Answer from the drawing. Dimensions are ordinates in mm from the lowest x, y and z of the part. Give positions to 0.01 mm unless a question says otherwise; leave off trailing zeros. Write each loop counter-clockwise with the first axis right and the second up, starting at its lowest first coordinate (ties: lowest second). Pieces come first, ordered by that corner, then holes. Notation, with made-up numbers: (62.25, 18) -> (103.25, 18) arc R8 ccw to (103.25, 31) -> close; hole circle Ø3 at (-1.75, 59). An arc over 180 degrees is marked (long way). Write item = value, one per line.
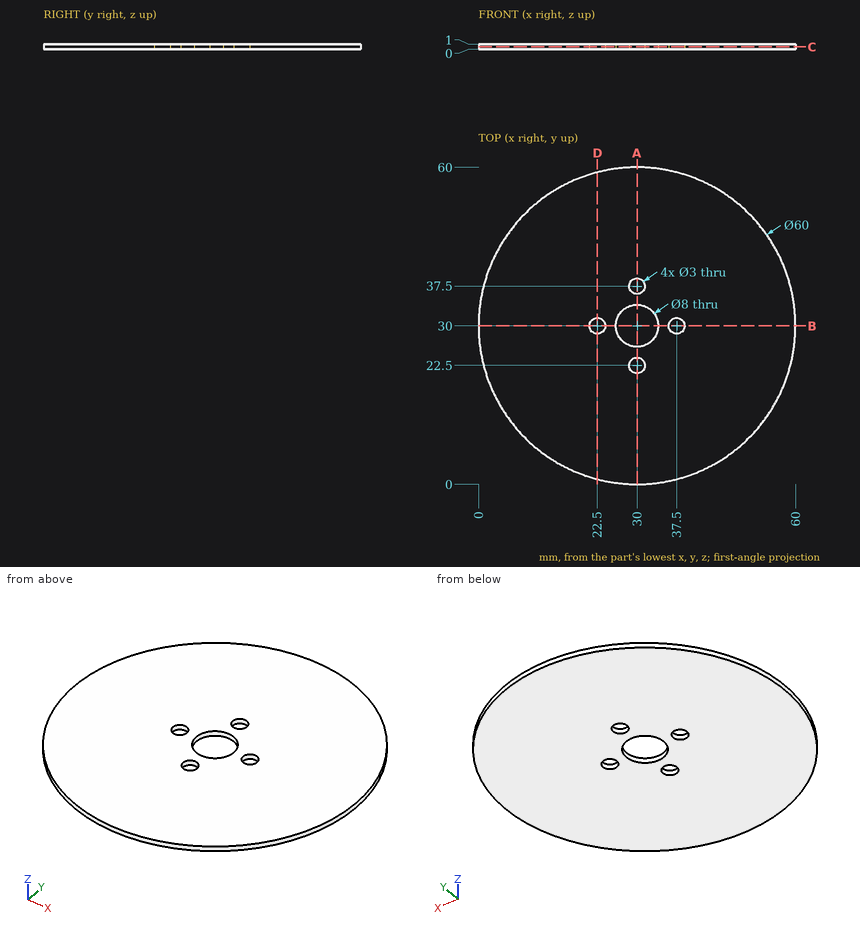
(1) The part is cut by section C-C on z = 0.45. Determine the outline of the cut face in (x, y).
Checks:
outline = circle Ø60 at (30, 30); hole circle Ø3 at (22.5, 30); hole circle Ø8 at (30, 30); hole circle Ø3 at (30, 22.5); hole circle Ø3 at (30, 37.5); hole circle Ø3 at (37.5, 30)
(2) The part is cut by section D-D on x = 22.5. Determine the outline of the cut face in (y, z).
Checks:
outline = (0.95, 0) -> (28.5, 0) -> (28.5, 1) -> (0.95, 1) -> close; (31.5, 0) -> (59.05, 0) -> (59.05, 1) -> (31.5, 1) -> close
(3) Given P1, Ø9, axis at x = 30, y = 30, coming from the +Z side, flat-ended and moving along its own axis, determine where the tip first touches the part or whether it passes through.
Checks:
P1 = 1
(4) Consider L1, parallel to Y at x = 30, z = 0.45; L2, parallel to X at y = 29, z = 0.25; L3, parallel to Y at x = 23.5, z = 0.95. Determine where each line is inside the solid, lowest interval first.
Checks:
L1 = 0 to 21, 24 to 26, 34 to 36, 39 to 60
L2 = 0.02 to 21.38, 23.62 to 26.13, 33.87 to 36.38, 38.62 to 59.98
L3 = 0.71 to 28.88, 31.12 to 59.29
(5) The part is cut by section A-A on x = 30. Determine the outline of the cut face in (y, z).
Checks:
outline = (0, 0) -> (21, 0) -> (21, 1) -> (0, 1) -> close; (24, 0) -> (26, 0) -> (26, 1) -> (24, 1) -> close; (34, 0) -> (36, 0) -> (36, 1) -> (34, 1) -> close; (39, 0) -> (60, 0) -> (60, 1) -> (39, 1) -> close
